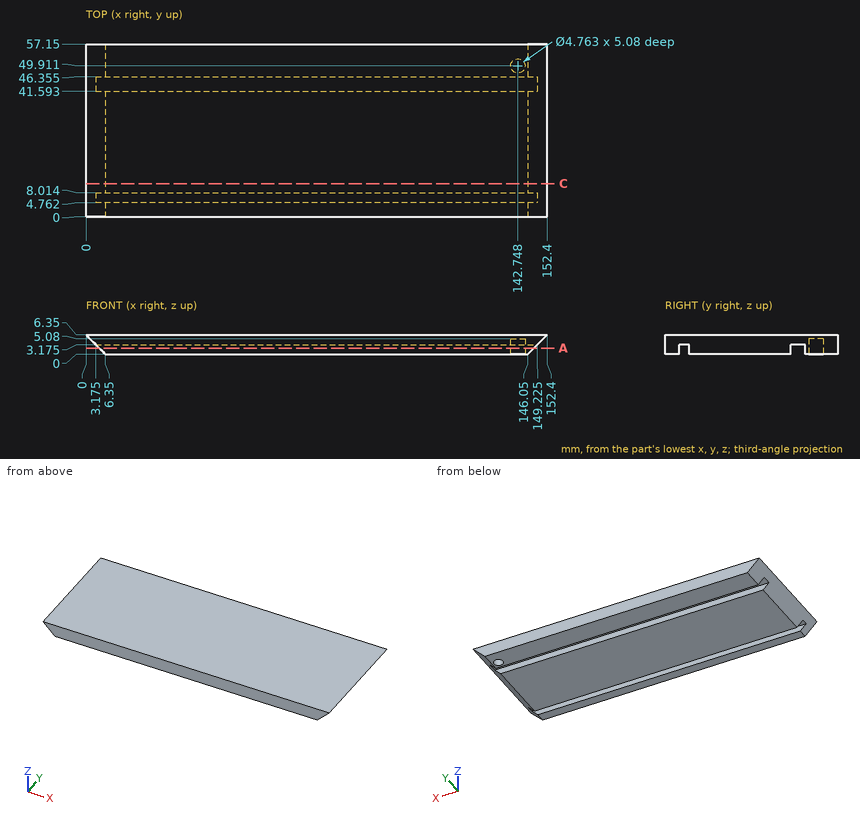
Print and shaded views of the part. All mm, measured from the part's lowest x, y and z. Coordinates: 2 decimals unless noted, no trailing zeros. Order: outer loops, then holes, each group sorted by start corner. A loop starts at its lowest first (then second) coordinate and runs counter-clockwise, first axis right, second up.
Item 1: Saw through at A-A on z = 2. State how many separate pieces and enclosed holes the cut face has, then the cut area to 3 significant figures.
Filled in:
separate pieces: 3
enclosed holes: 1
area: 7,040 mm2
Item 2: Drill centre lines: L1, parallel to X at y = 39, z = 5.5; L2, parallel to X at y = 41.5, z = 5.25. Where is each one in solid material? Low to high.
Filled in:
L1: x = 0.85 to 151.55
L2: x = 1.1 to 151.3
Item 3: Saw through at C-C on y = 11. List the corners of the cut face in (x, z).
Filled in:
outline: (0, 6.35) - (6.35, 0) - (146.05, 0) - (152.4, 6.35) - close
Item 4: Drop flat-ended pins along their axis: pin 1 Ø5.5 at (x, y) = (142.748, 49.911) entering from -Z; pin 2 Ø4 at (x, y) = (93, 44) entering from -Z (1 decimal). Give the stop position or say it passes through.
Filled in:
pin 1: stops at z = 0
pin 2: stops at z = 3.2
